Check sheet for the modelled part. Datum: model origin and axes. Units: mm. Face numbers are marked on the shaded views. Coordinates: 2 decimals unless noted, no trailing zeros. Loops run counter-clockwise (first coordinate to the right, second up) from the corner with the lowest first, then second, coordinate; pieces in that order, holes last. Notation, with made-up numbers: M 48,64 L 98,64 A30 ccw 98,91 Z; hole C 11,-37 d5. An arc over 180 degrees is marked long. Answer as CSV lines item,"result". Start each with the question number.
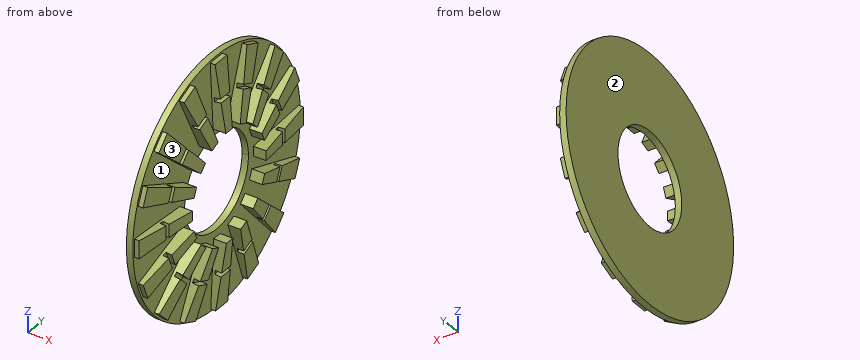
from build123d import *

# Parameters (mm, degrees)
F1_DEPTH    = 6
F2_W        = 6
F2_H        = 1.25
F3_DEPTH    = 2
F4_T1_DEPTH = 132.091103715
F6_COUNT    = 16
F5_R        = 38.75
F7_DEPTH    = 2


# Not quite as in the source:
# - a fillet or chamfer that OpenCascade refuses, or shapes differently, is made with other operations: its cross-section is extruded or revolved along the edge and cut away or added


with BuildPart() as f1:
    # F0 (on Front) → F1 (new body)
    with BuildSketch(Plane.XZ):
        Polygon((0, 21), (0, 0), (6, 0), (3.5, 21), align=None)
    extrude(amount=F1_DEPTH)

    # F2 (on face) → F3 (cut)
    with BuildSketch(Plane(origin=(5.9161542761, 0, 0.7043040805), x_dir=(0, 1, 0), z_dir=(0.9929882742, 0, 0.1182128898))):
        with Locations((-3, 9.2398656526)):
            Rectangle(F2_W, F2_H)
    extrude(amount=-F3_DEPTH, mode=Mode.SUBTRACT)

    # F4: chamfer of 1.5 x 24.25 on 2 edges, made by hand

    # F4_s2 → F4_t1 (cut)
    with BuildSketch(Plane.YZ.offset(-63.0455518575)):
        Polygon((-4.5, 0), (-6, 24.25), (-6, 0), align=None)
        Polygon((-1.5, 0), (0, 24.25), (0, 0), align=None)
    extrude(amount=F4_T1_DEPTH, mode=Mode.SUBTRACT)


with BuildPart() as f6_1:
    # F6: instance of F1
    add(f1.part.rotate(Axis((0, -2.8759991925, -16.9995477528), (1, 0, 0)), 1 * 360 / F6_COUNT))


with BuildPart() as f6_2:
    # F6: instance of F1
    add(f1.part.rotate(Axis((0, -2.8759991925, -16.9995477528), (1, 0, 0)), 2 * 360 / F6_COUNT))


with BuildPart() as f6_3:
    # F6: instance of F1
    add(f1.part.rotate(Axis((0, -2.8759991925, -16.9995477528), (1, 0, 0)), 3 * 360 / F6_COUNT))


with BuildPart() as f6_4:
    # F6: instance of F1
    add(f1.part.rotate(Axis((0, -2.8759991925, -16.9995477528), (1, 0, 0)), 4 * 360 / F6_COUNT))


with BuildPart() as f6_5:
    # F6: instance of F1
    add(f1.part.rotate(Axis((0, -2.8759991925, -16.9995477528), (1, 0, 0)), 5 * 360 / F6_COUNT))


with BuildPart() as f6_6:
    # F6: instance of F1
    add(f1.part.rotate(Axis((0, -2.8759991925, -16.9995477528), (1, 0, 0)), 6 * 360 / F6_COUNT))


with BuildPart() as f6_7:
    # F6: instance of F1
    add(f1.part.rotate(Axis((0, -2.8759991925, -16.9995477528), (1, 0, 0)), 7 * 360 / F6_COUNT))


with BuildPart() as f6_8:
    # F6: instance of F1
    add(f1.part.rotate(Axis((0, -2.8759991925, -16.9995477528), (1, 0, 0)), 8 * 360 / F6_COUNT))


with BuildPart() as f6_9:
    # F6: instance of F1
    add(f1.part.rotate(Axis((0, -2.8759991925, -16.9995477528), (1, 0, 0)), 9 * 360 / F6_COUNT))


with BuildPart() as f6_10:
    # F6: instance of F1
    add(f1.part.rotate(Axis((0, -2.8759991925, -16.9995477528), (1, 0, 0)), 10 * 360 / F6_COUNT))


with BuildPart() as f6_11:
    # F6: instance of F1
    add(f1.part.rotate(Axis((0, -2.8759991925, -16.9995477528), (1, 0, 0)), 11 * 360 / F6_COUNT))


with BuildPart() as f6_12:
    # F6: instance of F1
    add(f1.part.rotate(Axis((0, -2.8759991925, -16.9995477528), (1, 0, 0)), 12 * 360 / F6_COUNT))


with BuildPart() as f6_13:
    # F6: instance of F1
    add(f1.part.rotate(Axis((0, -2.8759991925, -16.9995477528), (1, 0, 0)), 13 * 360 / F6_COUNT))


with BuildPart() as f6_14:
    # F6: instance of F1
    add(f1.part.rotate(Axis((0, -2.8759991925, -16.9995477528), (1, 0, 0)), 14 * 360 / F6_COUNT))


with BuildPart() as f6_15:
    # F6: instance of F1
    add(f1.part.rotate(Axis((0, -2.8759991925, -16.9995477528), (1, 0, 0)), 15 * 360 / F6_COUNT))


with BuildPart() as f1_1:
    add(f1.part)

    add(f6_1.part)  # F7 merges F6_1

    add(f6_2.part)  # F7 merges F6_2

    add(f6_3.part)  # F7 merges F6_3

    add(f6_4.part)  # F7 merges F6_4

    add(f6_5.part)  # F7 merges F6_5

    add(f6_6.part)  # F7 merges F6_6

    add(f6_7.part)  # F7 merges F6_7

    add(f6_8.part)  # F7 merges F6_8

    add(f6_9.part)  # F7 merges F6_9

    add(f6_10.part)  # F7 merges F6_10

    add(f6_11.part)  # F7 merges F6_11

    add(f6_12.part)  # F7 merges F6_12

    add(f6_13.part)  # F7 merges F6_13

    add(f6_14.part)  # F7 merges F6_14

    add(f6_15.part)  # F7 merges F6_15
    # F5 (on Right) → F7 (join)
    with BuildSketch(Plane.YZ):
        with Locations((-2.8759991925, -16.9995477528)):
            Circle(F5_R)
        with BuildLine():
            ThreePointArc((-2.9835881284, -2.2499401438), (7.5157177781, -6.53175341), (11.8740008075, -16.9995477528))
            ThreePointArc((11.8740008075, -16.9995477528), (-13.2677161631, -27.4673420956), (-2.9835881284, -2.2499401438))
        make_face(mode=Mode.SUBTRACT)
    extrude(amount=F7_DEPTH)


solid = f1_1.part
Item 1: Sectioned sample at A-A, the plane y = 1. Record the boundary of the cut face in (x, z), and give its area (3 significant figures).
Item 2: Go/stop test with flat-tipped pins: pin 1 (2 mm diameter, centred on y = 19.5, z = -16.5, fed in from +X); pin 2 (1.5 mm diameter, centred on x = 3.5, z = -0.5, fed in from +Y); pin 3 (1.5 mm diameter, centred on x = 3, y = -2.5, fed in from -Z). Record where each tip stops, or that it passes through.
Item 3: Release check for a two-part mould opening along Z. For the marked faces 1, 2 and 3 record: released by +Z, released by -Z, zero draft, split by the parting line, or undercut.
Item 4: Material ranges on line 1 (Y direction, x = 2.5, z = -52); line 2 (Z direction, x = 5, y = -19); line 3 (Z direction, x = 2.75, y = 14.5) (3 decimals), recorded low to high. Write a range as from..to.
Item 5: Sectioned sample at B-B, the plane y = 30. Record the boundary of the cut face in (x, z), and give its area (3 significant figures).
Reply:
1,outline,"M 0,-55.56 L 2,-55.56 L 2,-31.23 L 0,-31.23 Z; M 0,-2.77 L 2,-2.77 L 2,21.56 L 0,21.56 Z"
1,area,"97.3 mm²"
2,pin 1,"x = 5.48"
2,pin 2,"y = 31.73"
2,pin 3,"z = -55"
3,face 1,"undercut"
3,face 2,"zero draft"
3,face 3,"released by +Z"
4,line 1,"-17.68..-14.3, -5.37..-0.14, 8.81..11.92"
4,line 2,"-36.11..-30.81, -25.51..-22.49, -11.5..-8.76, -3.52..1.74"
4,line 3,"-37.156..-31.589, -25.85..-22.365, -18.399..-15.352, -11.372..-7.874, -2.08..3.531"
5,outline,"M 0,-37.51 L 2,-37.51 L 2,-33.42 L 3.66,-33.42 L 3.92,-27.69 L 2,-27.69 L 2,-19.36 L 4.11,-19.36 L 4.11,-14.39 L 2,-14.39 L 2,-6.05 L 3.91,-6.05 L 3.65,-0.3 L 2,-0.3 L 2,3.51 L 0,3.51 Z"
5,area,"113 mm²"
